```python
from build123d import *

# Parameters (mm, degrees)
SKETCH1_R           = 3
BOSS_EXTRUDE1_DEPTH = 2
SKETCH2_R           = 2
BOSS_EXTRUDE2_DEPTH = 14
CUT_EXTRUDE2_DEPTH  = 1


with BuildPart() as part:
    # Sketch1 → Boss-Extrude1 (new body)
    with BuildSketch(Plane(origin=(0, 0, 0), x_dir=(1, 0, 0), z_dir=(0, 1, 0))):
        Circle(SKETCH1_R)
    extrude(amount=BOSS_EXTRUDE1_DEPTH)

    # Sketch2 → Boss-Extrude2 (add)
    with BuildSketch(Plane(origin=(0, 2, 0), x_dir=(1, 0, 0), z_dir=(0, 1, 0))):
        Circle(SKETCH2_R)
    extrude(amount=BOSS_EXTRUDE2_DEPTH)

    # Sketch3 → Cut-Extrude2 (cut)
    with BuildSketch(Plane.XZ):
        Polygon((0, 0.3), (3.344738487, 0.3), (3.344738487, 0), (3.344738487, -0.3), (0, -0.3), (-3.50820315, -0.3), (-3.50820315, 0), (-3.50820315, 0.3), align=None)
    extrude(amount=-CUT_EXTRUDE2_DEPTH, mode=Mode.SUBTRACT)


solid = part.part
```
The listing builds one solid part. Answer for the finished solid, in the listing's coordinates (mm). A direction names the side the tool comes from. Give positions to 0.01 mm unless a question says otherwise; leave off trailing zeros. Order: outer loops, then holes, each group sorted by start corner. A loop starts at its lowest first (then second) coordinate and runs counter-clockwise, first axis right, second up. Notation, with made-up numbers: (21.5, -28.75) -> (59.5, -28.75) arc R20 ccw to (59.5, -12.75) -> close; hole circle Ø1 at (41, 79.25). An arc over 180 degrees is marked (long way). Answer as a JSON object with one key per item and string values. Group by question number.
Item 1: The part is cut by section A-A on x = 0. Write down the section's boundary in (y, z), and give its area (3 significant figures).
Item 2: The part is cut by section C-C on y = 8.5. Write down the section's boundary in (x, z).
Item 3: The part is cut by section B-B on z = 0. Write down the section's boundary in (x, y), and give its area (3 significant figures).
Item 4: Determine the mould class of faces 4 (the flat face through (0, 0, 1)), 5 (the flat face through (0, 0.5, 0.3)), 6 (the cylindrical face through (0, 9, 2)) for opening direction Z: pulls with the +Z half, pulls with the -Z half, needs draft (parallel to the pull), parting line crosses it, or undercut.
Item 5: A tool of negligible diameter and unlimited length cuts with its end or side. For faces 1 (the flat face through (0, 0, -1)), 2 (the flat face through (0, 0.5, -0.3)), 3 (the flat face through (1, 2, 2)), from which of +Z, -Z, +X, -X, +Y, -Y can it reach the whole face along a straight path? Write none if from no direction.
Item 6: Flat-ended cylindrical pins translate along their axes: pin 1 (0.5 mm diameter, centred on x = 1, y = 0.5, fed in from +Z); pin 2 (3 mm diameter, centred on x = -1, y = 13.5, fed in from +Z); pin 3 (0.5 mm diameter, centred on x = -1.5, y = 0.5, fed in from -Z). Find the tip coordinate at first contact, or state that the pin passes through.
Item 7: The part is cut by section D-D on x = 1.1. Write down the section's boundary in (y, z), and give its area (3 significant figures).
Item 8: Consider L1, parallel to Y at x = 0.45, z = 2.2; L2, parallel to Y at x = 0.5, z = 0.1; L3, parallel to X at y = 12.5, z = -0.05. Determine where each line is inside the solid, lowest interval first. Write a range as from..to.
Result set:
{
 "1": {"outline": "(0, -3) -> (2, -3) -> (2, -2) -> (16, -2) -> (16, 2) -> (2, 2) -> (2, 3) -> (0, 3) -> (0, 0.3) -> (1, 0.3) -> (1, -0.3) -> (0, -0.3) -> close", "area": "67.4 mm²"},
 "2": {"outline": "circle Ø4 at (0, 0)"},
 "3": {"outline": "(-3, 1) -> (3, 1) -> (3, 2) -> (2, 2) -> (2, 16) -> (-2, 16) -> (-2, 2) -> (-3, 2) -> close", "area": "62.0 mm²"},
 "4": {"face 4": "needs draft", "face 5": "undercut", "face 6": "parting line crosses it"},
 "5": {"face 1": "+Z, -Z, +X, -X, -Y", "face 2": "+X, -X, -Y", "face 3": "+Y"},
 "6": {"pin 1": "z = 2.9", "pin 2": "z = 2", "pin 3": "z = -2.73"},
 "7": {"outline": "(0, -2.79) -> (2, -2.79) -> (2, -1.67) -> (16, -1.67) -> (16, 1.67) -> (2, 1.67) -> (2, 2.79) -> (0, 2.79) -> (0, 0.3) -> (1, 0.3) -> (1, -0.3) -> (0, -0.3) -> close", "area": "57.3 mm²"},
 "8": {"L1": "0..2", "L2": "1..16", "L3": "-2..2"}
}
